Work out the finished part from the listing and answer in its coordinate system (mm). A direction names the side the tool comes from. Round coordinates to 2 decimals unless told otherwise and drop trailing zeros. Write each loop counter-clockwise with the first axis right and the second up, starting at its lowest first coordinate (ties: lowest second). Pieces come first, ordered by that corner, then holes. Notation, with made-up numbers: M -10,32 L 7,32 A9 cw 7,46 Z; hole C 45.5,-29 d7. An arc over 180 degrees is marked long. Answer in a Markdown table with one row per item.
```python
from build123d import *

# Parameters (mm, degrees)
SKETCH1_W           = 266.7
SKETCH1_H           = 165.1
SKETCH1_W_2         = 254
SKETCH1_H_2         = 152.4
BOSS_EXTRUDE1_DEPTH = 215.9
SKETCH4_W           = 88.9
SKETCH4_H           = 165.1
CUT_EXTRUDE2_DEPTH  = 267.7
CUT_EXTRUDE3_REACH  = 167.1
SKETCH5_R           = 14.2875


with BuildPart() as part:
    # Sketch1 → Boss-Extrude1 (new body)
    with BuildSketch(Plane.XY):
        with Locations((133.35, 82.55)):
            Rectangle(SKETCH1_W, SKETCH1_H)
        with Locations((133.35, 82.55)):
            Rectangle(SKETCH1_W_2, SKETCH1_H_2, mode=Mode.SUBTRACT)
    extrude(amount=BOSS_EXTRUDE1_DEPTH)

    # Sketch4 → Cut-Extrude2 (cut, through all)
    with BuildSketch(Plane(origin=(266.7, 0, 0), x_dir=(0, 0, -1), z_dir=(1, 0, 0))):
        with Locations((-171.45, 82.55)):
            Rectangle(SKETCH4_W, SKETCH4_H)
    extrude(amount=-CUT_EXTRUDE2_DEPTH, mode=Mode.SUBTRACT)

    # Sketch5 → Cut-Extrude3 (cut, up to next)
    with BuildSketch(Plane(origin=(0, 165.1, 0), x_dir=(1, 0, 0), z_dir=(0, 1, 0)), mode=Mode.PRIVATE) as cut_extrude3_sk1:
        with Locations((133.35, -101.6)):
            Circle(SKETCH5_R)
    cut_extrude3_tool1 = extrude(cut_extrude3_sk1.sketch, amount=-CUT_EXTRUDE3_REACH, mode=Mode.PRIVATE) & part.part
    add(cut_extrude3_tool1.solids().sort_by_distance((133.35, 165.1, 101.6))[0], mode=Mode.SUBTRACT)


solid = part.part
```
1. Consider line 1 along Y through (x, z) = (70.5, 37); line 2 along Z through (x, y) = (133, 160); line 3 along X through (y, z) = (161, 101.6). Determine where each line is inside the solid, lowest interval first. Write a range as from..to.
Calculated:
| item | result |
|---|---|
| line 1 | y = 0..6.35, 158.75..165.1 |
| line 2 | z = 0..87.32, 115.88..127 |
| line 3 | x = 0..119.06, 147.64..266.7 |
2. The part is cut by section B-B (x = 32). Determine the outline of the cut face in (y, z), plus the area to 3 significant figures.
Calculated:
| item | result |
|---|---|
| outline | M 0,0 L 6.35,0 L 6.35,127 L 0,127 Z; M 158.75,0 L 165.1,0 L 165.1,127 L 158.75,127 Z |
| area | 1,610 mm² |
3. The part is cut by section D-D (x = 133.35). Determine the outline of the cut face in (y, z).
Calculated:
| item | result |
|---|---|
| outline | M 0,0 L 6.35,0 L 6.35,127 L 0,127 Z; M 158.75,0 L 165.1,0 L 165.1,87.31 L 158.75,87.31 Z; M 158.75,115.89 L 165.1,115.89 L 165.1,127 L 158.75,127 Z |
4. Determine the mould class of faces 4 (the flat face through (131, 0, 63)), 5 (the flat face through (0, 81, 63)), 6 (the flat face through (132, 158.75, 63)) for opening direction X: released by +X, released by -X, zero draft, split by the parting line, or undercut.
Calculated:
| item | result |
|---|---|
| face 4 | zero draft |
| face 5 | released by -X |
| face 6 | undercut |
5. A tool of negligible diameter and unlimited length cuts with its end or side. For faces 1 (the flat face through (132, 6.35, 63)), 2 (the cylindrical face through (139.943, 161.969, 114.275)), 3 (the flat face through (266.7, 81, 63)), from which of +Z, -Z, +X, -X, +Y, -Y can it reach the whole face along a straight path? Write none if from no direction.
Calculated:
| item | result |
|---|---|
| face 1 | +Z, -Z |
| face 2 | +Y |
| face 3 | +Z, -Z, +X, +Y, -Y |
6. The part is cut by section C-C (z = 101.6). Determine the outline of the cut face in (x, y).
Calculated:
| item | result |
|---|---|
| outline | M 0,0 L 266.7,0 L 266.7,165.1 L 147.64,165.1 L 147.64,158.75 L 260.35,158.75 L 260.35,6.35 L 6.35,6.35 L 6.35,158.75 L 119.06,158.75 L 119.06,165.1 L 0,165.1 Z |
7. The part is cut by section A-A (y = 133.5). Determine the outline of the cut face in (x, z), plus the area to 3 significant figures.
Calculated:
| item | result |
|---|---|
| outline | M 0,0 L 6.35,0 L 6.35,127 L 0,127 Z; M 260.35,0 L 266.7,0 L 266.7,127 L 260.35,127 Z |
| area | 1,610 mm² |
